```python
from build123d import *

# Parameters (mm, degrees)
BOSS_EXTRUDE1_DEPTH = 5
SKETCH3_R           = 15
BOSS_EXTRUDE2_DEPTH = 3


with BuildPart() as part:
    # Sketch1 → Boss-Extrude1 (new, symmetric)
    with BuildSketch(Plane.XY):
        with BuildLine():
            Line((-25, 0), (-25, 50))
            Line((-25, 50), (25, 50))
            Line((25, 50), (25, 0))
            ThreePointArc((25, 0), (0, -25), (-25, 0))
        make_face()
    extrude(amount=BOSS_EXTRUDE1_DEPTH, both=True)

    # Sketch3 → Boss-Extrude2 (add)
    with BuildSketch(Plane.XY.offset(5)):
        Circle(SKETCH3_R)
    extrude(amount=BOSS_EXTRUDE2_DEPTH)


solid = part.part
```
Geometry check sheet. Reference: the model listing, model coordinates, mm. A direction names the side the tool comes from. Coordinates: 2 decimals unless noted, no trailing zeros. Order: outer loops, then holes, each group sorted by start corner. A loop starts at its lowest first (then second) coordinate and runs counter-clockwise, first axis right, second up. Notation, with made-up numbers: (75.25, 15) - (112.25, 15) arc R17 ccw to (112.25, 35) - close; hole circle Ø5 at (1, 77.25). An arc over 180 degrees is marked (long way). Answer in a Markdown table with one row per item. Add a question column.
1. Section check B-B (y = -3). Enter the section's corners in (x, z).
2. Section check A-A (x = 0). Enter the section's corners in (y, z), plus the area to 3 significant figures.
3. Section check C-C (z = 4). Enter the section's corners in (x, y), plus the area to 3 significant figures.
4. Access from +Z, -Z, +X, -X, +Y, -Y to the whole of each face (thin tool, end or side, straight path). Record for faces 1 (the face through (-14.985, 0.66, 6.479)), 2 (the face through (0, 0, 8)).
5. Section check D-D (y = 38.5). Enter the section's corners in (x, z), plus the area to 3 significant figures.
6. Material ranges on L1, parallel to Z at x = 22.5, y = 3.5; L2, parallel to Y at x = 0, z = 0.5; L3, parallel to X at y = -0.5, z = 4 (3 decimals), recorded low to high. Write a range as [from, to].
Data:
| question | item | result |
|---|---|---|
| 1 | outline | (-24.82, -5) - (24.82, -5) - (24.82, 5) - (14.7, 5) - (14.7, 8) - (-14.7, 8) - (-14.7, 5) - (-24.82, 5) - close |
| 2 | outline | (-25, -5) - (50, -5) - (50, 5) - (15, 5) - (15, 8) - (-15, 8) - (-15, 5) - (-25, 5) - close |
| 2 | area | 840 mm² |
| 3 | outline | (-25, 0) arc R25 ccw to (25, 0) - (25, 50) - (-25, 50) - close |
| 3 | area | 3,480 mm² |
| 4 | face 1 | +Z |
| 4 | face 2 | +Z, +X, -X, +Y, -Y |
| 5 | outline | (-25, -5) - (25, -5) - (25, 5) - (-25, 5) - close |
| 5 | area | 500 mm² |
| 6 | L1 | z = [-5, 5] |
| 6 | L2 | y = [-25, 50] |
| 6 | L3 | x = [-24.995, 24.995] |
